CAD build for the part. Positions are in the model's coordinates, mm. Face numbers are marked on the shaded views. A direction names the side the tool comes from. Coordinates: 2 decimals unless noted, no trailing zeros. Loops run counter-clockwise (first coordinate to the right, second up) from the corner with the lowest first, then second, coordinate; pieces in that order, holes last.
1) Which spindle directions (+Z, -Z, +X, -X, +Y, -Y) get a long thin tool onto all of the face, cutting with end or side? Do the marked faces 5, 6 and 7. Say none if no direction does.
2) Saw through at D-D, the plane z = 4. Write the cut outline in (x, y) (3 decimals).
3) Wall check: line 1 along Y through (x, z) = (-1.5, -8); line 2 along Z through (x, y) = (2, 22.5) (3 decimals); line 3 along Z through (x, y) = (9, 7.5). Give the ranges that are in metal, low to high.
4) Two-plate mould, pull along X, no slides. Class the marked faces 1, 2, 3 and 4: +X half, -X half, draft (parallel to the pull), parting line (faces both ways), or undercut.
5) Saw through at C-C, the plane x = 0.5. Write the cut outline in (y, z) (3 decimals).
6) Saw through at B-B, the plane x = -8.5. Write the cut outline in (y, z) (3 decimals), and give its area (3 significant figures).
7) Saw through at A-A, the plane y = 22. Write the cut outline in (x, z) (3 decimals).
8) Pin check, flat tips, straight feed: pin 1 Ø3 at (y, z) = (13.5, -10) entering from -X; pin 2 Ø4 at (x, y) = (11, 10.5) entering from -Z; pin 3 Ø5.5 at (x, z) = (2.5, -1.5) entering from +Y. Stop position of each tip, or through.
Autodesk Inventor part; units mm, degrees
ref_plane "YZ Plane" through (0, 0, 0) normal (1, 0, 0) x (0, 1, 0)
ref_plane "XZ Plane" through (0, 0, 0) normal (0, 1, 0) x (-1, 0, 0)
ref_plane "XY Plane" through (0, 0, 0) normal (0, 0, 1) x (1, 0, 0)
sketch "Sketch1" plane through (0, 0, 0) normal (0, 1, 0) x (-1, 0, 0)
  line L0 (-12.7, -12.7) -> (-12.7, 12.7)
  line L1 (-12.7, 12.7) -> (12.7, 12.7)
  line L2 (12.7, 12.7) -> (12.7, -12.7)
  line L3 (12.7, -12.7) -> (-12.7, -12.7)
  point P0 (0, 0)
  point P1 (0, 0)
  dimension "d0" = 25.4
extrude "Extrusion1" add sketch "Sketch1" along normal blind 25.4
sketch "Sketch2" plane through (0, 25.4, 0) normal (0, 1, 0) x (1, 0, 0)
  line L0 (9.525, 9.525) -> (9.525, -9.525)
  line L1 (9.525, -9.525) -> (-9.525, -9.525)
  line L2 (-9.525, -9.525) -> (-9.525, 9.525)
  line L3 (-9.525, 9.525) -> (9.525, 9.525)
  point P0 (0, 0)
  point P1 (0, 0)
  dimension "d3" = 19.05
extrude "Extrusion2" cut sketch "Sketch2" against normal blind 5
sketch "Sketch3" plane through (12.7, 0, 12.7) normal (1, 0, 0) x (0, 0, -1)
  line L0 (22.225, 20.4) -> (3.175, 20.4)
  line L1 (17.7, 7.4) -> (7.7, 7.4)
  line L2 (7.7, 7.4) -> (7.7, 17.4)
  line L3 (7.7, 17.4) -> (17.7, 17.4)
  line L4 (17.7, 17.4) -> (17.7, 7.4)
  point P0 (12.7, 0)
  point P1 (12.7, 12.4)
  dimension "d6" = 10
extrude "Extrusion3" cut sketch "Sketch3" against normal blind 5
pattern_circular "Circular Pattern1" count 4 over 360 about axis through (0, -10, 0) along (0, 1, 0) of "Extrusion3"
sketch "Sketch4" plane through (0, 0, 0) normal (0, -1, 0) x (1, 0, 0)
  line L0 (12.7, -12.7) -> (12.7, 12.7)
  line L1 (12.7, 12.7) -> (-12.7, 12.7)
  line L2 (-12.7, 12.7) -> (-12.7, -12.7)
  line L3 (-12.7, -12.7) -> (12.7, -12.7)
  point P0 (0, 0)
extrude "Extrusion4" add sketch "Sketch4" along normal blind 15 draft 45
properties part number "frame_nexus_2_base"
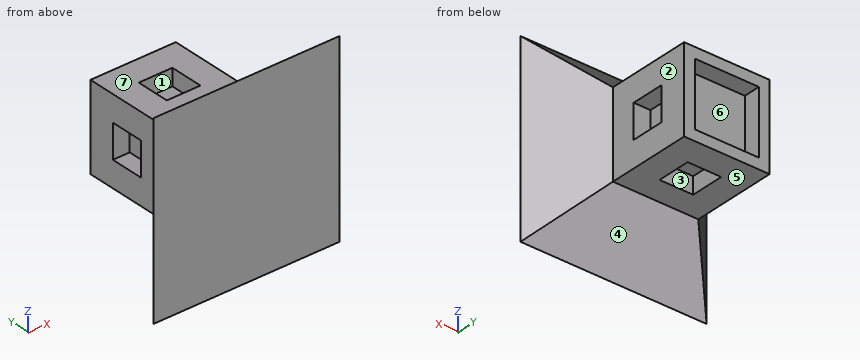
Data:
1. face 5: -Z, +X, -X, +Y
1. face 6: +Y
1. face 7: +Z, +X, -X, +Y
2. outline: (-27.7, -15) - (27.7, -15) - (12.7, 0) - (12.7, 7.4) - (7.7, 7.4) - (7.7, 17.4) - (12.7, 17.4) - (12.7, 25.4) - (9.525, 25.4) - (9.525, 20.4) - (-9.525, 20.4) - (-9.525, 25.4) - (-12.7, 25.4) - (-12.7, 17.4) - (-7.7, 17.4) - (-7.7, 7.4) - (-12.7, 7.4) - (-12.7, 0) - close
3. line 1: y = -15 to 7.4, 17.4 to 20.4
3. line 2: z = -12.7 to -9.525, 9.525 to 12.7
3. line 3: z = -12.7 to -5, 5 to 12.7
4. face 1: undercut
4. face 2: +X half
4. face 3: undercut
4. face 4: draft
5. outline: (-15, -27.7) - (0, -12.7) - (7.4, -12.7) - (7.4, -7.7) - (17.4, -7.7) - (17.4, -12.7) - (25.4, -12.7) - (25.4, -9.525) - (20.4, -9.525) - (20.4, 9.525) - (25.4, 9.525) - (25.4, 12.7) - (17.4, 12.7) - (17.4, 7.7) - (7.4, 7.7) - (7.4, 12.7) - (0, 12.7) - (-15, 27.7) - close
6. outline: (-15, -27.7) - (0, -12.7) - (25.4, -12.7) - (25.4, -9.525) - (20.4, -9.525) - (20.4, 9.525) - (25.4, 9.525) - (25.4, 12.7) - (0, 12.7) - (-15, 27.7) - close; hole (7.4, -5) - (17.4, -5) - (17.4, 5) - (7.4, 5) - close
6. area: 1,060 mm2
7. outline: (-12.7, -12.7) - (12.7, -12.7) - (12.7, 12.7) - (-12.7, 12.7) - close; hole (-9.525, -9.525) - (9.525, -9.525) - (9.525, 9.525) - (-9.525, 9.525) - close
8. pin 1: stops at x = -12.7
8. pin 2: stops at z = -12.7
8. pin 3: stops at y = 20.4
